Autodesk Inventor part; units mm, degrees
ref_plane "YZ Plane" through (0, 0, 0) normal (1, 0, 0) x (0, 1, 0)
ref_plane "XZ Plane" through (0, 0, 0) normal (0, 1, 0) x (-1, 0, 0)
ref_plane "XY Plane" through (0, 0, 0) normal (0, 0, 1) x (1, 0, 0)
sketch "Sketch1" plane through (0, 0, 0) normal (0, 1, 0) x (-1, 0, 0)
  line L0 (0, 0) -> (120, 0)
  line L1 (120, 0) -> (120, -180)
  line L2 (120, -180) -> (0, -180)
  line L3 (0, -180) -> (0, 0)
  dimension "d0" = 120
  dimension "d1" = 180
extrude "Extrusion1" add sketch "Sketch1" along normal blind 2
sketch "Sketch2" plane through (0, 2, 0) normal (0, 1, 0) x (1, 0, 0)
  line L0 (-120, 0) -> (0, 0)
  line L1 (0, 0) -> (-8, 0)
  line L2 (-8, 0) -> (-8, 8)
  line L3 (-8, 8) -> (0, 8)
  line L4 (0, 8) -> (0, 0)
  line L5 (-120, 180) -> (-120, 0)
  line L6 (-120, 90) -> (0, 90)
  line L7 (0, 0) -> (0, 180)
  line L8 (-60, 0) -> (-60, 180)
  line L9 (0, 180) -> (-120, 180)
  line L10 (0, 180) -> (-8, 180)
  line L11 (-8, 180) -> (-8, 172)
  line L12 (-8, 172) -> (0, 172)
  line L13 (0, 172) -> (0, 180)
  line L14 (-120, 0) -> (-112, 0)
  line L15 (-112, 0) -> (-112, 8)
  line L16 (-112, 8) -> (-120, 8)
  line L17 (-120, 8) -> (-120, 0)
  line L18 (-120, 180) -> (-112, 180)
  line L19 (-112, 180) -> (-112, 172)
  line L20 (-112, 172) -> (-120, 172)
  line L21 (-120, 172) -> (-120, 180)
  line L22 (-120, 8) -> (-118, 8)
  line L23 (-118, 8) -> (-118, 172)
  line L24 (-118, 172) -> (-120, 172)
  line L25 (-120, 172) -> (-120, 8)
  line L26 (0, 172) -> (-2, 172)
  line L27 (-2, 172) -> (-2, 8)
  line L28 (-2, 8) -> (0, 8)
  line L29 (0, 8) -> (0, 172)
  line L30 (-8, 0) -> (-112, 0)
  line L31 (-112, 0) -> (-112, 2)
  line L32 (-112, 2) -> (-8, 2)
  line L33 (-8, 2) -> (-8, 0)
  line L34 (-8, 180) -> (-112, 180)
  line L35 (-112, 180) -> (-112, 178)
  line L36 (-112, 178) -> (-8, 178)
  line L37 (-8, 178) -> (-8, 180)
  point P0 (-8, 2)
  point P1 (-8, 178)
  dimension "d4" = 8
  dimension "d5" = 8
  dimension "d10" = 2
  dimension "d12" = 2
  dimension "d13" = 2
  dimension "d21" = 2
extrude "Extrusion2" add sketch "Sketch2" along normal blind 45 contours L15 L32 L8 L0 | L5 L6 L23 L16 | L8 L32 L2 L0 | L5 L20 L23 L6 | L3 L27 L6 L7 | L27 L12 L7 L6 | L36 L19 L9 L8 | L8 L9 L11 L36
sketch "Sketch4" plane through (0, 2, 0) normal (0, 1, 0) x (1, 0, 0)
  line L0 (0, 0) -> (-4, 0)
  line L1 (-4, 0) -> (-4, 4)
  line L2 (-4, 4) -> (0, 4)
  line L3 (0, 4) -> (0, 0)
  circle A0 centre (-4, 4) radius 1.5
  line L4 (-120, 180) -> (-120, 0)
  line L5 (-120, 90) -> (0, 90)
  line L6 (0, 8) -> (0, 180)
  line L7 (-120, 0) -> (0, 0)
  line L8 (-60, 0) -> (-60, 180)
  line L9 (0, 180) -> (-120, 180)
  circle A1 centre (-4, 176) radius 1.5
  circle A2 centre (-116, 4) radius 1.5
  circle A3 centre (-116, 176) radius 1.5
  point P0 (-120, 172)
  point P1 (-120, 8)
  point P2 (0, 172)
  dimension "d16" = 4
  dimension "d17" = 4
  dimension "d18" = 3
extrude "Extrusion3" cut sketch "Sketch4" against normal blind 45 contours A0 L2 L1 | L1 L2 A0 | A1 | A2 | A3
fillet "Fillet1" radius 3 4 edges at (-120, 1, -180) (0, 1, -180) (-120, 1, 0) (0, 1, 0)
properties part number "reduced_tortoise_base"
Part model, mm, in its own coordinate system. A direction names the side the tool comes from. Give positions to 0.01 mm unless a question says otherwise; leave off trailing zeros. Order: outer loops, then holes, each group sorted by start corner. A loop starts at its lowest first (then second) coordinate and runs counter-clockwise, first axis right, second up. Notation, with made-up numbers: (85.25, -22.5) - (128.25, -22.5) arc R22 ccw to (128.25, -13.5) - close; hole circle Ø1 at (13.25, -19). An arc over 180 degrees is marked (long way). One line per question, with ' | ' between items.
1. Drop flat-ended pins along their axis: P1, Ø3, axis at x = -69.5, z = -96, coming from the +Y side; P2, Ø1, axis at x = -119.5, y = 24, coming from the +Z side; P3, Ø0.6, axis at y = 22.5, z = -179.5, coming from the +X side. Give the stop position or say it passes through.
Filled in:
P1: y = 2 | P2: z = -8 | P3: x = -8
2. Which spindle directions (+Z, -Z, +X, -X, +Y, -Y) get a long thin tool onto all of the face, cutting with end or side? Do faces 1 (the face through (-2, 24, -91)), 2 (the face through (-61, 24, -178)), 3 (the face through (-120, 23, -89)). Say none if no direction does.
Filled in:
face 1: +Z, -Z, +Y | face 2: +X, -X, +Y | face 3: +Z, -Z, -X, +Y, -Y
3. Band-saw the part on C-C on x = -68. List the corners of the cut face in (y, z), then the cut area to 3 significant figures.
Filled in:
outline: (0, -180) - (47, -180) - (47, -178) - (2, -178) - (2, -2) - (47, -2) - (47, 0) - (0, 0) - close | area: 540 mm²
4. Drill centre lines: probe 1 along X at (y, z) = (1.35, -176); probe 2 along Z at (x, y) = (-116, 1); probe 3 along X at (y, z) = (18.5, -52.5). Where is each one in solid material? Low to high.
Filled in:
probe 1: -120 to -117.5, -114.5 to -5.5, -2.5 to 0 | probe 2: -180 to -177.5, -174.5 to -5.5, -2.5 to 0 | probe 3: -120 to -118, -2 to 0
5. Band-saw the part on A-A on y = 37. List the corners of the cut face in (x, z), then the cut area to 3 significant figures.
Filled in:
outline: (-120, -172) - (-118, -172) - (-118, -8) - (-120, -8) - close; (-112, -180) - (-8, -180) - (-8, -178) - (-112, -178) - close; (-112, -2) - (-8, -2) - (-8, 0) - (-112, 0) - close; (-2, -172) - (0, -172) - (0, -8) - (-2, -8) - close | area: 1,070 mm²
6. Pull direction X, two halves, no side cores. Call faces 4 (the face through (-118, 24, -89)), 5 (the face through (0, 23, -91)), 6 (the face through (-59, 0, -89)): +X half, -X half, draft (parallel to the pull), parting line (faces both ways), or undercut.
Filled in:
face 4: undercut | face 5: +X half | face 6: draft
7. Band-saw the part on B-B on z = -116. List the corners of the cut face in (x, y), then the cut area to 3 significant figures.
Filled in:
outline: (-120, 0) - (0, 0) - (0, 47) - (-2, 47) - (-2, 2) - (-118, 2) - (-118, 47) - (-120, 47) - close | area: 420 mm²
